Can you work these out from the drawing? Everything is in mm from the part's minimum corner. Give positions to 0.01 mm unless a question says otherwise; leave off trailing zeros. Order: outer loops, then holes, each group sorted by start corner. A loop starts at its lowest first (then second) coordinate and runs counter-clockwise, first axis right, second up. Notation, with made-up numbers: M -23,31 L 25,31 A21 ccw 25,70 Z; hole C -4,-13 d11. An arc over 180 degrees is marked long. Answer as a JSON object with one key per item and string values.
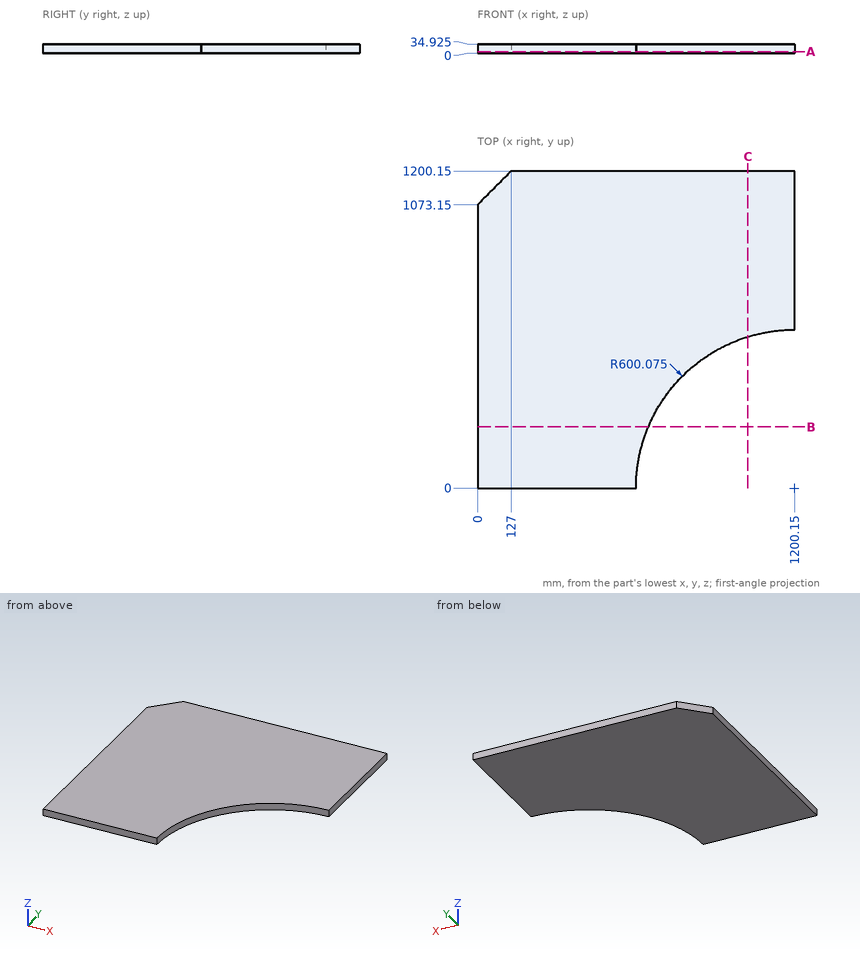
1) I want a section at B-B on y = 232. Write out the boundary of the cut face in (x, z) (3 decimals), and give its area (3 significant figures).
Results found:
{"outline": "M 0,0 L 646.737,0 L 646.737,34.925 L 0,34.925 Z", "area": "22,600 mm²"}
2) I need wall thicknesses on L1, parallel to Y at x = 86.5, z = 23; L2, parallel to Y at x = 1140.5, z = 16.5; L3, parallel to X at y = 422, z = 11.5. Which ranges of each line are inside material? Lowest first, please.
Results found:
{"L1": "y = 0 to 1159.65", "L2": "y = 597.1 to 1200.15", "L3": "x = 0 to 773.53"}
3) I'm going to push a flat-ended pin straight in: pin 1 Ø6 at (x, z) = (973.5, 6.5) entering from -Y. Where does the tip first touch, or does it pass through?
Results found:
{"pin 1": "stops at y = 554.39"}
4) I want a section at A-A on z = 6. Write out the boundary of the cut face in (x, y) (3 decimals), and give its area (3 significant figures).
Results found:
{"outline": "M 0,0 L 600.075,0 A600.075 cw 1200.15,600.075 L 1200.15,1200.15 L 127,1200.15 L 0,1073.15 Z", "area": "1,150,000 mm²"}
5) I want a section at C-C on x = 1024. Write out the boundary of the cut face in (y, z) (3 decimals), and give its area (3 significant figures).
Results found:
{"outline": "M 573.639,0 L 1200.15,0 L 1200.15,34.925 L 573.639,34.925 Z", "area": "21,900 mm²"}
